```python
from build123d import *

# Parameters (mm, degrees)
SKETCH_W        = 95
SKETCH_H        = 74
PAD_DEPTH       = 5
SKETCH002_W     = 72
SKETCH002_H     = 40
POCKET_DEPTH    = 5.001
SKETCH004_W     = 117.661896
SKETCH004_H     = 92.433091
SKETCH004_W_2   = 80
SKETCH004_H_2   = 53
POCKET001_DEPTH = 3
FILLET_R        = 3
FILLET001_R     = 3
SKETCH005_R     = 3
POCKET002_DEPTH = 5
SKETCH006_W     = 5.477936
SKETCH006_H     = 50
SKETCH006_W_2   = 5.931454
POCKET003_DEPTH = 5
FILLET002_R     = 1


with BuildPart() as part:
    # Sketch → Pad (new body)
    with BuildSketch(Plane.XY):
        Rectangle(SKETCH_W, SKETCH_H)
    extrude(amount=PAD_DEPTH)

    # Sketch002 → Pocket (cut, through all)
    with BuildSketch(Plane.XY.offset(5)):
        Rectangle(SKETCH002_W, SKETCH002_H)
    extrude(amount=-POCKET_DEPTH, mode=Mode.SUBTRACT)

    # Sketch004 → Pocket001 (cut)
    with BuildSketch(Plane.XY.offset(5)):
        with Locations((-1.857784, 0.611237)):
            Rectangle(SKETCH004_W, SKETCH004_H)
        Rectangle(SKETCH004_W_2, SKETCH004_H_2, mode=Mode.SUBTRACT)
    extrude(amount=-POCKET001_DEPTH, mode=Mode.SUBTRACT)

    # Fillet
    fillet_edges = [part.edges().sort_by_distance(p)[0] for p in [
        (-36, 20, 2.5),
        (36, 20, 2.5),
        (36, -20, 2.5),
        (-36, -20, 2.5),
    ]]
    fillet(fillet_edges, radius=FILLET_R)

    # Fillet001
    fillet001_edges = [part.edges().sort_by_distance(p)[0] for p in [
        (40, 26.5, 3.5),
        (47.5, 37, 1),
        (47.5, -37, 1),
        (40, -26.5, 3.5),
        (-47.5, -37, 1),
        (-40, -26.5, 3.5),
        (-40, 26.5, 3.5),
        (-47.5, 37, 1),
    ]]
    fillet(fillet001_edges, radius=FILLET001_R)

    # Sketch005 → Pocket002 (cut)
    with BuildSketch(Plane.XY.offset(2)):
        with Locations((-44, 32.5)):
            Circle(SKETCH005_R)
        with Locations((44, 32.5)):
            Circle(SKETCH005_R)
        with Locations((44, -32.5)):
            Circle(SKETCH005_R)
        with Locations((-44, -32.5)):
            Circle(SKETCH005_R)
    extrude(amount=-POCKET002_DEPTH, mode=Mode.SUBTRACT)

    # Sketch006 → Pocket003 (cut)
    with BuildSketch(Plane.XY.offset(2)):
        with Locations((46.738968, 0)):
            Rectangle(SKETCH006_W, SKETCH006_H)
        with Locations((-46.965727, 0)):
            Rectangle(SKETCH006_W_2, SKETCH006_H)
    extrude(amount=-POCKET003_DEPTH, mode=Mode.SUBTRACT)

    # Fillet002
    fillet002_edges = [part.edges().sort_by_distance(p)[0] for p in [
        (-47.5, 25, 1),
        (-44, 25, 1),
        (-44, -25, 1),
        (-47.5, -25, 1),
        (47.5, -25, 1),
        (44, -25, 1),
        (44, 25, 1),
        (47.5, 25, 1),
    ]]
    fillet(fillet002_edges, radius=FILLET002_R)


solid = part.part
```
Design review of the part built by this model. Coordinates are the model's own, in mm. A direction names the side the tool comes from. Round coordinates to 2 decimals unless told otherwise and drop trailing zeros. Order: outer loops, then holes, each group sorted by start corner. A loop starts at its lowest first (then second) coordinate and runs counter-clockwise, first axis right, second up. Notation, with made-up numbers: (41, 31) - (60, 31) arc R25 ccw to (60, 60) - close; hole circle Ø7 at (89, 29). An arc over 180 degrees is marked (long way). Return JSON: item names as keys, results as strings.
Q1. Wall thickness on L1, parallel to Y at x = 17, z = 1.1; L2, parallel to X at y = -12, z = 3.5; L3, parallel to Y at x = 26.5, z = 2.95: over which ranges is each line inside the solid? List them lowest first. Write a range as [from, to].
Computed values:
{"L1": "y = [-37, -20], [20, 37]", "L2": "x = [-40, -36], [36, 40]", "L3": "y = [-26.5, -20], [20, 26.5]"}
Q2. The part is to be moulded in two halves that separate along Y. For faces 1 (the flat face through (47.5, -30, 1)), 2 (the flat face through (0, -20, 3)), 3 (the flat face through (-1, -37, 1)), say which applies: pulls with the +Y half, pulls with the -Y half, needs draft (parallel to the pull), parting line crosses it, or undercut.
Computed values:
{"face 1": "needs draft", "face 2": "undercut", "face 3": "pulls with the -Y half"}
Q3. Consider section B-B on x = -30.5. Write out the cut boundary in (y, z).
Computed values:
{"outline": "(-37, 0) - (-20, 0) - (-20, 5) - (-26.5, 5) - (-26.5, 2) - (-37, 2) - close; (20, 0) - (37, 0) - (37, 2) - (26.5, 2) - (26.5, 5) - (20, 5) - close"}
Q4. Machinability: for faces 4 (the flat face through (-1, 26.5, 4)), 5 (the cylindrical face through (39.1, 25.64, 3.48)), 6 (the cylindrical face through (35.1, -19.14, 2.46)), 7 (the flat face through (-40, 0, 4)), which of the approach directions +Z, -Z, +X, -X, +Y, -Y give a long, thin tool a straight path to every point of the face, cutting with its end or side? Answer none if there is none.
Computed values:
{"face 4": "+Z, +X, -X, +Y", "face 5": "+Z, +X, +Y", "face 6": "+Z, -Z", "face 7": "+Z, -X, +Y, -Y"}
Q5. Consider section D-D on y = 32.5. Write out the cut boundary in (x, z), plus the area to 3 significant figures.
Computed values:
{"outline": "(-47.5, 0) - (-47, 0) - (-47, 2) - (-47.5, 2) - close; (-41, 0) - (41, 0) - (41, 2) - (-41, 2) - close; (47, 0) - (47.5, 0) - (47.5, 2) - (47, 2) - close", "area": "166 mm2"}
Q6. Consider section C-C on z = 3.05. Write out the cut boundary in (x, y), plus the area to 3 significant figures.
Computed values:
{"outline": "(-40, -23.5) arc R3 ccw to (-37, -26.5) - (37, -26.5) arc R3 ccw to (40, -23.5) - (40, 23.5) arc R3 ccw to (37, 26.5) - (-37, 26.5) arc R3 ccw to (-40, 23.5) - close; hole (-36, -17) arc R3 ccw to (-33, -20) - (33, -20) arc R3 ccw to (36, -17) - (36, 17) arc R3 ccw to (33, 20) - (-33, 20) arc R3 ccw to (-36, 17) - close", "area": "1,360 mm2"}
Q7. Consider section A-A on y = 6. Write out the cut boundary in (x, z).
Computed values:
{"outline": "(-44, 0) - (-36, 0) - (-36, 5) - (-40, 5) - (-40, 2) - (-44, 2) - close; (36, 0) - (44, 0) - (44, 2) - (40, 2) - (40, 5) - (36, 5) - close"}
Q8. For pin 1 Ø0.9 at (x, z) = (-11.5, 3.5) entering from +Y; pin 2 Ø1.5 at (y, z) = (17.5, 2.5) entering from +X; pin 3 Ø2.5 at (y, z) = (-8, 1.5) entering from -X, all flat-tipped, find the tip position at first contact; note any pin that passes through.
Computed values:
{"pin 1": "stops at y = 26.5", "pin 2": "stops at x = 44", "pin 3": "stops at x = -44"}
